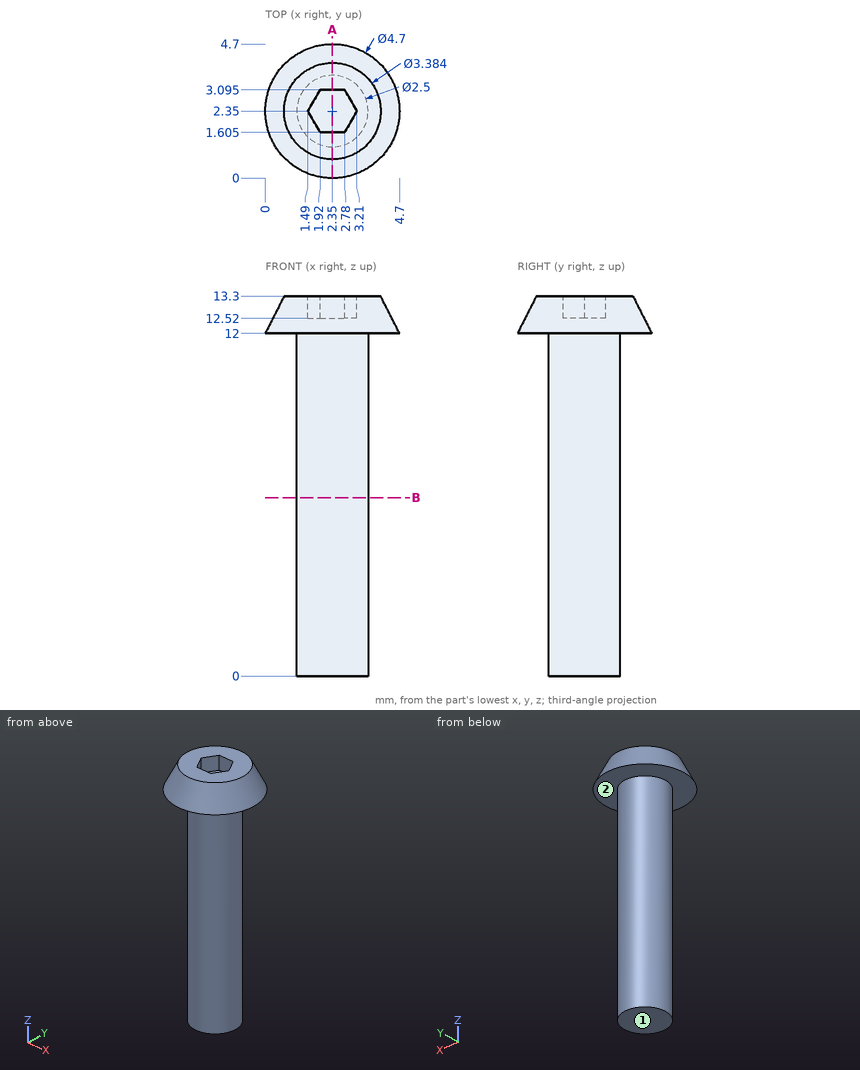
Input: dimensioned drawing with shaded views. Units: mm. Origin: part minimum x, y, z. A direction names the side the tool comes from. Coordinates: 2 decimals unless noted, no trailing zeros. Order: outer loops, then holes, each group sorted by start corner. A loop starts at its lowest first (then second) coordinate and runs counter-clockwise, first axis right, second up.
(1) Section query B-B (z = 6.25). Return the cut outline in (x, y).
(2) Access query for the marked faces 1 and 2. Directions: +Z, -Z, +X, -X, +Y, -Y. A direction counts if a zero-diameter tool reaches every point of the face in a straight line with its end or side. Return the directions, or none.
(3) First-contact query: pin 1 (1.5 mm diameter, centred on y = 1, z = 4.5, fed in from +X). Flat tip, straight axial feed; report the tip coordinate or a pass-through.
(4) Material intervals for probe 1 along Z at (x, y) = (1.15, 1.45); probe 2 along Y at (x, z) = (2.3, 11.5); probe 3 along Z at (x, y) = (1.45, 4.05), sorted ascending.
(5) Section query A-A (x = 2.35). Return the cut outline in (y, z) (1 decimal), plus the area to 3 significant figures.
Solution:
1. outline: circle Ø2.5 at (2.35, 2.35)
2. face 1: -Z, +X, -X, +Y, -Y
2. face 2: -Z
3. pin 1: stops at x = 3.45
4. probe 1: z = 12 to 13.3
4. probe 2: y = 1.1 to 3.6
4. probe 3: z = 12 to 12.84
5. outline: (0, 12) - (1.1, 12) - (1.1, 0) - (3.6, 0) - (3.6, 12) - (4.7, 12) - (4, 13.3) - (3.1, 13.3) - (3.1, 12.5) - (1.6, 12.5) - (1.6, 13.3) - (0.7, 13.3) - close
5. area: 34.1 mm2
